from build123d import *

# Parameters (mm, degrees)
F0_R     = 50
F1_DEPTH = 54.864
F3_DEPTH = 50.546


with BuildPart() as f1:
    # F0 (on Top) → F1 (new body)
    with BuildSketch(Plane.XY):
        Circle(F0_R)
    extrude(amount=F1_DEPTH)

    # F2 (on face) → F3 (join)
    with BuildSketch(Plane(origin=(0, 0, 0), x_dir=(1, 0, 0), z_dir=(0, 0, -1))):
        with BuildLine():
            Line((30.2700951576, 39.7959965216), (1.3566113452, 61.7885079781))
            Line((1.3566113452, 61.7885079781), (-28.494267061, 41.0862111256))
            ThreePointArc((-28.494267061, 41.0862111256), (1.0975221129, 49.9879530008), (30.2700951576, 39.7959965216))
        make_face()
        with BuildLine():
            Line((59.1835791051, 17.8034849624), (30.2700951576, 39.7959965216))
            ThreePointArc((30.2700951576, 39.7959965216), (44.7967898285, 22.209178757), (50, 0))
            ThreePointArc((50, 0), (49.2955920393, -8.3632891551), (47.2022157803, -16.4909316118))
            Line((47.2022157803, -16.4909316118), (59.1835791051, 17.8034849624))
        make_face()
        with BuildLine():
            ThreePointArc((50, 0), (44.7967898285, 22.209178757), (30.2700951576, 39.7959965216))
            ThreePointArc((30.2700951576, 39.7959965216), (1.0975221129, 49.9879530008), (-28.494267061, 41.0862111256))
            ThreePointArc((-28.494267061, 41.0862111256), (-47.2022150962, 16.49093357), (-47.8805218829, -14.4033199027))
            ThreePointArc((-47.8805218829, -14.4033199027), (-30.2700960741, -39.7959958245), (-1.097521687, -49.9879530102))
            ThreePointArc((-1.097521687, -49.9879530102), (28.4942681078, -41.0862103996), (47.2022157803, -16.4909316118))
            ThreePointArc((47.2022157803, -16.4909316118), (49.2955920393, -8.3632891551), (50, 0))
        make_face()
        with BuildLine():
            ThreePointArc((-47.8805218829, -14.4033199027), (-47.2022150962, 16.49093357), (-28.494267061, 41.0862111256))
            Line((-28.494267061, 41.0862111256), (-58.3451471843, 20.3839130822))
            Line((-58.3451471843, 20.3839130822), (-47.8805218829, -14.4033199027))
        make_face()
        with BuildLine():
            ThreePointArc((-1.097521687, -49.9879530102), (-30.2700960741, -39.7959958245), (-47.8805218829, -14.4033199027))
            Line((-47.8805218829, -14.4033199027), (-37.4158953837, -49.1905568696))
            Line((-37.4158953837, -49.1905568696), (-1.097521687, -49.9879530102))
        make_face()
        with BuildLine():
            Line((35.2208521177, -50.7853491531), (47.2022157803, -16.4909316118))
            ThreePointArc((47.2022157803, -16.4909316118), (28.4942681078, -41.0862103996), (-1.097521687, -49.9879530102))
            Line((-1.097521687, -49.9879530102), (35.2208521177, -50.7853491531))
        make_face()
    extrude(amount=F3_DEPTH)


solid = f1.part
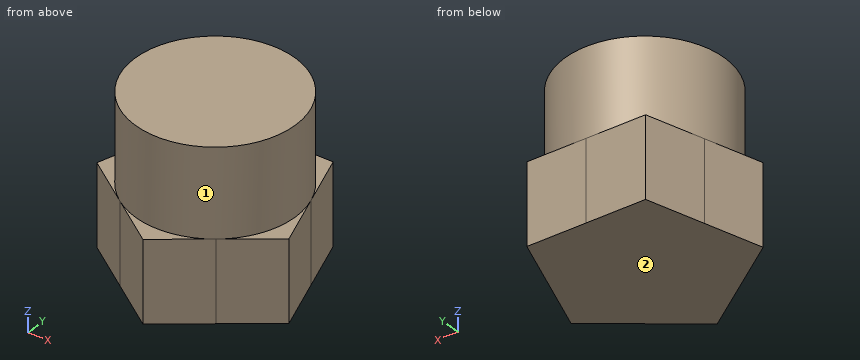
Design review of the part built by this model. Coordinates are the model's own, in mm. Face numbers are marked on the shaded views. A direction names the side the tool comes from. Give positions to 0.01 mm unless a question says otherwise; leave off trailing zeros. Loops run counter-clockwise (first coordinate to the right, second up) from the corner with the lowest first, then second, coordinate; pieces in that order, holes last. Notation, with made-up numbers: M -32,71 L 27,71 A15 ccw 27,99 Z; hole C 7,-35.75 d3. An arc over 180 degrees is marked long. One line per question, with ' | ' between items. Start each with the question number.
1. For the marked faces 1 and 2, list the 3-axis set-ups (+Z, -Z, +X, -X, +Y, -Y) from which the entire face can be reached by the end or side of a thin tool; tool diameter is ignored.
2. Add section B-B (x = 9). Write out the cut boundary in (y, z).
3. Insertion check: P1, Ø5, axis at x = 22, z = -1, coming from the +Y side; P2, Ø8, axis at x = 5, z = -18.5, coming from the +Y side; P3, Ø1, axis at y = 12, z = -13.5, coming from the +X side. Each pin has a flat end and moves straight along its axis. Give the tip position at first contact, or say it passes through.
4. To check wall thickness, follow L1, parallel to Z at x = -41, y = 30; L2, parallel to Y at x = -26.5, z = 47; L3, parallel to X at y = -48, z = -45. State the ranges of each line that lie inside material, in increasing order.
5. Add section C-C (y = 11). Write out the cut boundary in (x, z) (3 decimals), plus the area to 3 significant figures.
6. Add section A-A (z = -41.5). Write out the cut boundary in (x, y), plus the area to 3 significant figures.
7. Add section D-D (z = 16.5). Write out the cut boundary in (x, y), plus the area to 3 significant figures.
Worked out:
1) face 1: +Z | face 2: -Z, +X, -X, +Y, -Y
2) outline: M -55.97,-50.55 L 50.21,-50.55 L 50.21,0 L 49.18,0 L 49.18,54.86 L -49.18,54.86 L -49.18,0 L -55.97,0 Z
3) P1: stops at y = 50.55 | P2: stops at y = 50.21 | P3: stops at x = 48.95
4) L1: z = -50.55 to 0 | L2: y = -42.4 to 42.4 | L3: x = -18.53 to 19.48
5) outline: M -48.904,-50.546 L 49.121,-50.546 L 49.121,0 L 48.775,0 L 48.775,54.864 L -48.775,54.864 L -48.775,0 L -48.904,0 Z | area: 10,300 mm²
6) outline: M -58.35,-20.38 L 1.36,-61.79 L 59.18,-17.8 L 35.22,50.79 L -37.42,49.19 Z | area: 9,080 mm²
7) outline: C 0,0 d100 | area: 7,850 mm²
